The model under review builds one solid part; all positions refer to its coordinate system, in mm. A direction names the side the tool comes from. Coordinates: 2 decimals unless noted, no trailing zeros. Order: outer loops, then holes, each group sorted by start corner. A loop starts at its lowest first (then second) coordinate and runs counter-clockwise, first axis right, second up. Notation, with made-up numbers: (1.5, 23.25) -> (52.5, 23.25) arc R18 cw to (52.5, 48.25) -> close; hole circle Ø5 at (34, 66). An arc over 180 degrees is marked (long way). Put each result on its own line as item: value.
from build123d import *

# Parameters (mm, degrees)
SKETCH_1_R          = 24
EXTRUDE_1_DEPTH     = 10
SKETCH_2_R          = 14
EXTRUDE_2_DEPTH     = 40
SKETCH_3_R          = 8
CUT_EXTRUDE_1_DEPTH = 50
CUT_EXTRUDE_2_DEPTH = 10
SKETCH_5_R          = 3
SKETCH_5_R_2        = 2.542834368
SKETCH_5_R_3        = 3.082379743
SKETCH_5_R_4        = 2.48129437
SKETCH_5_R_5        = 2.732701735
CUT_EXTRUDE_3_DEPTH = 10


with BuildPart() as part:
    # 草图1 → 凸台-拉伸1 (new body)
    with BuildSketch(Plane.XY):
        Circle(SKETCH_1_R)
    extrude(amount=EXTRUDE_1_DEPTH)

    # 草图2 → 凸台-拉伸2 (add)
    with BuildSketch(Plane.XY.offset(10)):
        Circle(SKETCH_2_R)
    extrude(amount=EXTRUDE_2_DEPTH)

    # 草图3 → 切除-拉伸1 (cut)
    with BuildSketch(Plane.XY.offset(50)):
        Circle(SKETCH_3_R)
    extrude(amount=-CUT_EXTRUDE_1_DEPTH, mode=Mode.SUBTRACT)

    # 草图4 → 切除-拉伸2 (cut)
    with BuildSketch(Plane(origin=(0, 0, 0), x_dir=(-1, 0, 0), z_dir=(0, 0, -1))):
        with BuildLine():
            Line((-20, 13.266499161), (-20, -13.266499161))
            ThreePointArc((-20, -13.266499161), (-24, 0), (-20, 13.266499161))
        make_face()
        with BuildLine():
            Line((20, 13.266499161), (20, -13.266499161))
            ThreePointArc((20, -13.266499161), (24, 0), (20, 13.266499161))
        make_face()
    extrude(amount=-CUT_EXTRUDE_2_DEPTH, mode=Mode.SUBTRACT)

    # 草图5 → 切除-拉伸3 (cut)
    with BuildSketch(Plane(origin=(0, 0, 0), x_dir=(-1, 0, 0), z_dir=(0, 0, -1))):
        with Locations((0, 18.503142877)):
            Circle(SKETCH_5_R)
        with Locations((-13.083697802, -13.083697802)):
            Circle(SKETCH_5_R_2)
        with Locations((13.083697802, -13.083697802)):
            Circle(SKETCH_5_R_3)
        with Locations((13.083697802, 13.083697802)):
            Circle(SKETCH_5_R_4)
        with Locations((-13.083697802, 13.083697802)):
            Circle(SKETCH_5_R_5)
        with Locations((0, -18.503142877)):
            Circle(SKETCH_5_R)
    extrude(amount=-CUT_EXTRUDE_3_DEPTH, mode=Mode.SUBTRACT)


solid = part.part
Item 1: Consider section D-D on z = 20.5. Write out the cut boundary in (x, y), and give its area (3 significant figures).
Answers below:
outline: circle Ø28 at (0, 0); hole circle Ø16 at (0, 0)
area: 415 mm^2
Item 2: Consider section B-B on y = 5.5. Write out the cut boundary in (x, z).
Answers below:
outline: (-20, 0) -> (-5.81, 0) -> (-5.81, 50) -> (-12.87, 50) -> (-12.87, 10) -> (-20, 10) -> close; (5.81, 0) -> (20, 0) -> (20, 10) -> (12.87, 10) -> (12.87, 50) -> (5.81, 50) -> close
Item 3: Mouldability with a two-part tool opening along Y and no side actions: class faces 3 (the flat face through (20, 0, 5)), 4 (the cylindrical face through (0.391, 21.478, 4.93)), 5 (the cylindrical face through (0, 24, 5)) as +Y half, -Y half, draft (parallel to the pull), parting line (faces both ways), or undercut.
Answers below:
face 3: draft
face 4: undercut
face 5: +Y half
Item 4: Consider section C-C on z = 6. Write out the cut boundary in (x, y) (1 decimal).
Answers below:
outline: (-20, -13.3) arc R24 ccw to (20, -13.3) -> (20, 13.3) arc R24 ccw to (-20, 13.3) -> close; hole circle Ø6.2 at (-13.1, -13.1); hole circle Ø5 at (-13.1, 13.1); hole circle Ø16 at (0, 0); hole circle Ø6 at (0, -18.5); hole circle Ø6 at (0, 18.5); hole circle Ø5.5 at (13.1, 13.1); hole circle Ø5.1 at (13.1, -13.1)
Item 5: For line 1 (Z direction, x = 16, y = 15); line 2 (X direction, y = 0.5, z = 9); line 3 (Y direction, x = 0, z = 32), list the stretches that pass through material, from the lowest coordinate up. Write a range as from..to.
Answers below:
line 1: 0..10
line 2: -20..-7.98, 7.98..20
line 3: -14..-8, 8..14
Item 6: For pin 1 Ø8 at (y, z) = (7, 35) entering from +X; pin 2 Ø1.5 at (x, z) = (13, 10.5) entering from -Y; pin 3 Ø4 at (x, y) = (13.08, -13.08) entering from -Z; pin 4 Ø5 at (y, z) = (2.5, 37) entering from +X, all flat-tipped, find the tip position at first contact; note any pin that passes through.
Answers below:
pin 1: x = 13.67
pin 2: y = -20.52
pin 3: through
pin 4: x = 14
Item 7: Consider section A-A on x = 0. Write out the cut boundary in (y, z).
Answers below:
outline: (-24, 0) -> (-21.5, 0) -> (-21.5, 10) -> (-24, 10) -> close; (-15.5, 0) -> (-8, 0) -> (-8, 50) -> (-14, 50) -> (-14, 10) -> (-15.5, 10) -> close; (8, 0) -> (15.5, 0) -> (15.5, 10) -> (14, 10) -> (14, 50) -> (8, 50) -> close; (21.5, 0) -> (24, 0) -> (24, 10) -> (21.5, 10) -> close
Item 8: For faces 1 (the cylindrical face through (12.932, -5.362, 29.72)), 2 (the cylindrical face through (-12.682, -10.028, 4.93)), list the 3-axis set-ups (+Z, -Z, +X, -X, +Y, -Y) from which the entire face can be reached by the end or side of a thin tool; tool diameter is ignored.
Answers below:
face 1: +Z
face 2: +Z, -Z
